from build123d import *

# Parameters (mm, degrees)
SKETCH1_W               = 38.1
SKETCH1_H               = 76.2
BOSS_EXTRUDE1_DEPTH     = 76.2
SKETCH2_W               = 6.35
SKETCH2_H               = 50.8
CUT_EXTRUDE1_DEPTH      = 94.3255592
F_1_4_CLEARANCE_HOLE1_D = 6.7564
F_3_8_CLEARANCE_HOLE1_D = 10.0838
SKETCH7_R               = 4.7625
CUT_EXTRUDE2_DEPTH      = 94.3255592


with BuildPart() as part:
    # Sketch1 → Boss-Extrude1 (new body)
    with BuildSketch(Plane(origin=(0, 0, 0), x_dir=(1, 0, 0), z_dir=(0, 1, 0))):
        with Locations((-19.05, 0)):
            Rectangle(SKETCH1_W, SKETCH1_H)
    extrude(amount=BOSS_EXTRUDE1_DEPTH)

    # Sketch2 → Cut-Extrude1 (cut, through all)
    with BuildSketch(Plane(origin=(0, 76.2, 0), x_dir=(1, 0, 0), z_dir=(0, 1, 0))):
        with Locations((-3.175, 0)):
            Rectangle(SKETCH2_W, SKETCH2_H)
    extrude(amount=-CUT_EXTRUDE1_DEPTH, mode=Mode.SUBTRACT)

    # 1/4 Clearance Hole1 (through all)
    with Locations(Plane(origin=(0, 0, 0), x_dir=(0, 0, -1), z_dir=(1, 0, 0))):
        with Locations((0, 50.8), (0, 25.4), (-25.4, 25.4), (-25.4, 50.8), (25.4, 50.8), (25.4, 25.4)):
            Hole(F_1_4_CLEARANCE_HOLE1_D / 2)

    # 3/8 Clearance Hole1 (through all)
    with Locations(Plane(origin=(0, 76.2, 0), x_dir=(1, 0, 0), z_dir=(0, 1, 0))):
        with Locations((-22.225, -12.7), (-22.225, 12.7)):
            Hole(F_3_8_CLEARANCE_HOLE1_D / 2)

    # Sketch7 → Cut-Extrude2 (cut, through all)
    with BuildSketch(Plane(origin=(0, 76.2, 0), x_dir=(1, 0, 0), z_dir=(0, 1, 0))):
        with Locations((-6.35, 12.7)):
            Circle(SKETCH7_R)
        with Locations((-6.35, -12.7)):
            Circle(SKETCH7_R)
    extrude(amount=-CUT_EXTRUDE2_DEPTH, mode=Mode.SUBTRACT)


solid = part.part
Here's how the part is built. I have some questions about the finished solid (model axes, mm). A direction names the side the tool comes from. Coordinates: 2 decimals unless noted, no trailing zeros. Order: outer loops, then holes, each group sorted by start corner. A loop starts at its lowest first (then second) coordinate and runs counter-clockwise, first axis right, second up. Notation, with made-up numbers: (28, -8) -> (47, -8) arc R20 cw to (47, 25) -> close; hole circle Ø2 at (50, -9). An arc over 180 degrees is marked (long way). Answer in a Markdown table with one row per item.
(1) I want a section at D-D on x = -32. List the corners of the cut face in (y, z) for me.
Answer key:
| item | result |
|---|---|
| outline | (0, -38.1) -> (76.2, -38.1) -> (76.2, 38.1) -> (0, 38.1) -> close; hole circle Ø6.76 at (25.4, -25.4); hole circle Ø6.76 at (25.4, 0); hole circle Ø6.76 at (25.4, 25.4); hole circle Ø6.76 at (50.8, -25.4); hole circle Ø6.76 at (50.8, 0); hole circle Ø6.76 at (50.8, 25.4) |
(2) I want a section at A-A on x = -22. Count the separate pieces of the cut face and the enclosed holes in it, then the cut area to 3 significant figures.
Answer key:
| item | result |
|---|---|
| separate pieces | 3 |
| enclosed holes | 6 |
| area | 4,060 mm^2 |
(3) On a 3-axis mill with a long thin cutter (end or side, diameter ignored), from which of +Z, -Z, +X, -X, +Y, -Y can I reach the whole of each face in a straight line? I mean faces 1 (the face through (-3, 38, 25.4)), 2 (the face through (0, 38, -32)). Say none if no direction works.
Answer key:
| item | result |
|---|---|
| face 1 | +X, +Y, -Y |
| face 2 | +Z, -Z, +X, +Y, -Y |
(4) Thinking about a two-plate mould opening in Y: for faces 3 (the face through (-11.11, 38.63, 12.6)), 4 (the face through (-19, 0, -1)), 5 (the face through (-22.45, 54.15, -0.44)), which applies, +Y half, -Y half, draft (parallel to the pull), parting line (faces both ways), or undercut?
Answer key:
| item | result |
|---|---|
| face 3 | draft |
| face 4 | -Y half |
| face 5 | undercut |
(5) I want a section at C-C on z = -23.5. List the corners of the cut face in (x, y) for me, then the cut area to 3 significant figures.
Answer key:
| item | result |
|---|---|
| outline | (-38.1, 0) -> (-6.35, 0) -> (-6.35, 22.61) -> (-38.1, 22.61) -> close; (-38.1, 28.19) -> (-6.35, 28.19) -> (-6.35, 48.01) -> (-38.1, 48.01) -> close; (-38.1, 53.59) -> (-6.35, 53.59) -> (-6.35, 76.2) -> (-38.1, 76.2) -> close |
| area | 2,060 mm^2 |
(6) Please list where these lines run through material, in increasing order: probe 1 along Y at (x, z) = (-28, 0); probe 2 along Z at (x, y) = (-22, 18); probe 3 along X at (y, z) = (64, -13).
Answer key:
| item | result |
|---|---|
| probe 1 | 0 to 22.02, 28.78 to 47.42, 54.18 to 76.2 |
| probe 2 | -38.1 to -17.74, -7.66 to 7.66, 17.74 to 38.1 |
| probe 3 | -38.1 to -27.26, -17.19 to -11.1 |
(7) Will these pins go through, and if not, where does the flat tip stop? pin 1 Ø6.5 at (y, z) = (25.5, -21.5) entering from +X; pin 2 Ø11.5 at (x, z) = (-22.225, 12.7) entering from +Y.
Answer key:
| item | result |
|---|---|
| pin 1 | x = -6.35 |
| pin 2 | y = 76.2 |
